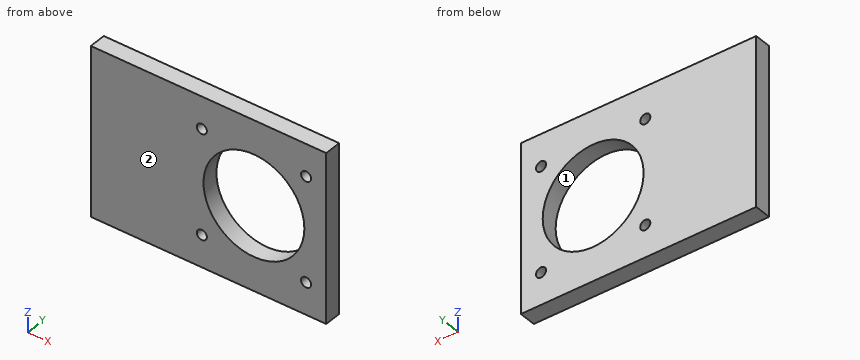
from build123d import *

# Parameters (mm, degrees)
SKETCH1_W           = 70
SKETCH1_H           = 50
BOSS_EXTRUDE1_DEPTH = 5
SKETCH2_R           = 1.5
CUT_EXTRUDE1_DEPTH  = 5
SKETCH3_R           = 15
CUT_EXTRUDE2_DEPTH  = 5


with BuildPart() as part:
    # Sketch1 → Boss-Extrude1 (new body)
    with BuildSketch(Plane(origin=(0, 0, 0), x_dir=(1, 0, 0), z_dir=(0, 1, 0))):
        Rectangle(SKETCH1_W, SKETCH1_H)
    extrude(amount=BOSS_EXTRUDE1_DEPTH)

    # Sketch2 → Cut-Extrude1 (cut)
    with BuildSketch(Plane(origin=(0, 5, 0), x_dir=(1, 0, 0), z_dir=(0, 1, 0))):
        with Locations((29, 15.5)):
            Circle(SKETCH2_R)
        with Locations((-2, 15.5)):
            Circle(SKETCH2_R)
    cut_extrude1 = extrude(amount=-CUT_EXTRUDE1_DEPTH, mode=Mode.SUBTRACT)

    # Mirror1: Cut-Extrude1 across plane
    add(cut_extrude1.mirror(Plane.XY), mode=Mode.SUBTRACT)

    # Sketch3 → Cut-Extrude2 (cut)
    with BuildSketch(Plane(origin=(0, 5, 0), x_dir=(1, 0, 0), z_dir=(0, 1, 0))):
        with Locations((13.5, 0)):
            Circle(SKETCH3_R)
    extrude(amount=-CUT_EXTRUDE2_DEPTH, mode=Mode.SUBTRACT)


solid = part.part
Geometry check sheet. Reference: the model listing, model coordinates, mm. Face numbers are marked on the shaded views. Round coordinates to 2 decimals unless told otherwise and drop trailing zeros. Loops run counter-clockwise (first coordinate to the right, second up) from the corner with the lowest first, then second, coordinate; pieces in that order, holes last.
Item 1: Gauge pin test, flat end, axial feed: pin 1 (12 mm diameter, centred on x = -21, z = -13.5, fed in from -Y). Record the tip position at first contact, or that the pin passes through.
Item 2: Cross-section at A-A on x = 13.5. Record the boundary of the cut face in (y, z).
Item 3: Cross-section at B-B on y = 1.15. Record the boundary of the cut face in (x, z).
Item 4: Cross-section at C-C on z = 0. Record the boundary of the cut face in (x, y), then the cut area to 3 significant figures.
Item 5: Thickness scan on line 1 (Z direction, x = 29, y = 3.65); line 2 (X direction, y = 1.8, z = -15.5); line 3 (Z direction, x = 13.5, y = 3.25). Record the ranges inside material, lowest first.
Item 6: Mould release check, pull along Z, two halves, no side actions. Record for the marked faces 1 and 2: pulls with the +Z half, pulls with the -Z half, needs draft (parallel to the pull), parting line crosses it, or undercut.
Answer sheet:
1. pin 1: stops at y = 0
2. outline: (0, -25) - (5, -25) - (5, -15) - (0, -15) - close; (0, 15) - (5, 15) - (5, 25) - (0, 25) - close
3. outline: (-35, -25) - (35, -25) - (35, 25) - (-35, 25) - close; hole circle Ø3 at (-2, -15.5); hole circle Ø3 at (-2, 15.5); hole circle Ø30 at (13.5, 0); hole circle Ø3 at (29, -15.5); hole circle Ø3 at (29, 15.5)
4. outline: (-35, 0) - (-1.5, 0) - (-1.5, 5) - (-35, 5) - close; (28.5, 0) - (35, 0) - (35, 5) - (28.5, 5) - close
4. area: 200 mm2
5. line 1: z = -25 to -17, -14 to 14, 17 to 25
5. line 2: x = -35 to -3.5, -0.5 to 27.5, 30.5 to 35
5. line 3: z = -25 to -15, 15 to 25
6. face 1: undercut
6. face 2: needs draft
